from build123d import *

# Parameters (mm, degrees)
F1_DEPTH = 25.4
F2_W     = 9.046357
F2_H     = 3.819572
F3_DEPTH = 25.4


with BuildPart() as f1:
    # F0 (on Front) → F1 (new body)
    with BuildSketch(Plane.XZ):
        Polygon((0, 27.641645), (0, 0), (26.435465, 0), (26.435465, 9.548932), (11.358204, 9.548932), (11.358204, 27.641645), align=None)
    extrude(amount=F1_DEPTH)

    # F2 (on face) → F3 (cut)
    with BuildSketch(Plane.YZ.offset(11.358204)):
        with Locations((-12.262839, 25.731859)):
            Rectangle(F2_W, F2_H)
    extrude(amount=-F3_DEPTH, mode=Mode.SUBTRACT)


solid = f1.part
Source: CAD feature listing. Evaluate the final solid. Frame: model axes, mm. A direction names the side the tool comes from. Coordinates: 2 decimals unless noted, no trailing zeros. Loops run counter-clockwise (first coordinate to the right, second up) from the corner with the lowest first, then second, coordinate; pieces in that order, holes last. Notation, with made-up numbers: (17, 19) - (36, 19) arc R28 cw to (36, 46) - close; hole circle Ø1 at (35.5, -40). An arc over 180 degrees is marked (long way). Return JSON: item names as keys, results as strings.
Q1. Access query for faces 1 (the flat face through (6, -12, 23.822)), 2 (the flat face through (11.358, -13, 18)), 3 (the flat face through (10, -25.4, 11)). Directions: +Z, -Z, +X, -X, +Y, -Y. A direction counts if a zero-diameter tool reaches every point of the face in a straight line with its end or side. Return the directions, or none.
Results:
{"face 1": "+Z, +X, -X", "face 2": "+Z, +X, +Y, -Y", "face 3": "+Z, -Z, +X, -X, -Y"}
Q2. Section A-A, the plane z = 24.25. Return loops of the section in (x, y).
Results:
{"outline": "(0, -25.4) - (11.36, -25.4) - (11.36, -16.79) - (0, -16.79) - close; (0, -7.74) - (11.36, -7.74) - (11.36, 0) - (0, 0) - close"}
Q3. Material intervals for line 1 along Y through (x, z) = (7, 26); line 2 along X through (y, z) = (-2.75, 20); line 3 along Z through (x, y) = (22.5, -4.5), sorted ascending.
Results:
{"line 1": "-25.4 to -16.79, -7.74 to 0", "line 2": "0 to 11.36", "line 3": "0 to 9.55"}
Q4. Section C-C, the plane x = 10.75. Return loops of the section in (y, z).
Results:
{"outline": "(-25.4, 0) - (0, 0) - (0, 27.64) - (-7.74, 27.64) - (-7.74, 23.82) - (-16.79, 23.82) - (-16.79, 27.64) - (-25.4, 27.64) - close"}
Q5. Section D-D, the plane y = -24. Return loops of the section in (x, z), plus the area to 3 significant figures.
Results:
{"outline": "(0, 0) - (26.44, 0) - (26.44, 9.55) - (11.36, 9.55) - (11.36, 27.64) - (0, 27.64) - close", "area": "458 mm2"}
Q6. Mould query, pull axis Y, two halves, no side actions, for faces 4 (the flat face through (6, -16.786, 26)), 5 (the flat face through (13, -13, 0)), 6 (the flat face through (10, 0, 11)). Classes: released by +Y, released by -Y, zero draft, split by the parting line, or undercut.
Results:
{"face 4": "undercut", "face 5": "zero draft", "face 6": "released by +Y"}
Q7. Contact query for flat-ended pins moving along their axis: P1, Ø5, axis at y = -12, z = 21.5, coming from the +X side; P2, Ø1, axis at x = 4.5, y = -13.5, coming from the +Z side; P3, Ø12, axis at x = 19, y = -9.5, coming from the +Z side. Output: stop coordinate, or through.
Results:
{"P1": "x = 11.36", "P2": "z = 23.82", "P3": "z = 9.55"}
Q8. Section B-B, the plane y = -10. Return loops of the section in (x, z).
Results:
{"outline": "(0, 0) - (26.44, 0) - (26.44, 9.55) - (11.36, 9.55) - (11.36, 23.82) - (0, 23.82) - close"}
